Build history of the part. All positions in model axes, mm. Round coordinates to 2 decimals unless told otherwise and drop trailing zeros. Loops run counter-clockwise (first coordinate to the right, second up) from the corner with the lowest first, then second, coordinate; pieces in that order, holes last. Notation, with made-up numbers: (18, -37.75) -> (25, -37.75) arc R18 ccw to (25, -28.75) -> close; hole circle Ø9 at (36, 2.5). An arc over 180 degrees is marked (long way). Put each result on its own line as item: value. Start each with the question number.
```python
from build123d import *

# Parameters (mm, degrees)
SKETCH2_W           = 90
SKETCH2_H           = 94.61
SKETCH2_R           = 1.5
BOSS_EXTRUDE1_DEPTH = 3
SKETCH3_W           = 10.64
SKETCH3_H           = 65.81
CUT_EXTRUDE1_DEPTH  = 10
CHAMFER1_SIZE       = 2


with BuildPart() as part:
    # Sketch2 → Boss-Extrude1 (new body)
    with BuildSketch(Plane(origin=(0, 0, 0), x_dir=(1, 0, 0), z_dir=(0, 1, 0))):
        Rectangle(SKETCH2_W, SKETCH2_H)
        with Locations((40.082878696, -39.905)):
            Circle(SKETCH2_R, mode=Mode.SUBTRACT)
        with Locations((-40.357121304, -39.905)):
            Circle(SKETCH2_R, mode=Mode.SUBTRACT)
        with Locations((40.082878696, 40.095)):
            Circle(SKETCH2_R, mode=Mode.SUBTRACT)
        with Locations((-40.357121304, 40.095)):
            Circle(SKETCH2_R, mode=Mode.SUBTRACT)
    extrude(amount=BOSS_EXTRUDE1_DEPTH)

    # Sketch3 → Cut-Extrude1 (cut)
    with BuildSketch(Plane(origin=(0, 0, 0), x_dir=(-1, 0, 0), z_dir=(0, -1, 0))):
        with Locations((39.68, 0)):
            Rectangle(SKETCH3_W, SKETCH3_H)
        with Locations((-39.68, 0)):
            Rectangle(SKETCH3_W, SKETCH3_H)
    extrude(amount=-CUT_EXTRUDE1_DEPTH, mode=Mode.SUBTRACT)

    # Chamfer1
    chamfer1_edges = [part.edges().sort_by_distance(p)[0] for p in [
        (0, 0, -47.305),
    ]]
    chamfer(chamfer1_edges, length=CHAMFER1_SIZE)


solid = part.part
```
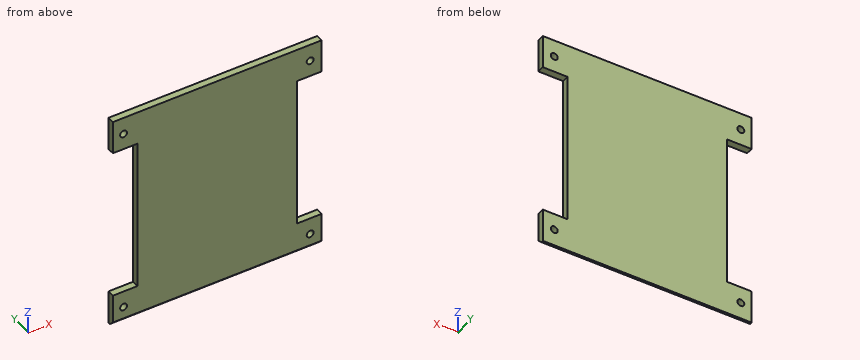
Item 1: Drop a flat-ended pin along its axis: pin 1 (1.5 mm diameter, centred on y = 2, z = 8, fed in from -X). Give the stop position or say it passes through.
Item 2: Cut at A-A on y = 0.9. Write the cut outline in (x, z) (3 decimals), then the cut area to 3 significant figures.
Item 3: Cut at B-B on z = -28.5. Write the cut outline in (x, y).
Item 4: Wall check: line 1 (Z direction, x = 35.5, y = 2.55) (3 decimals); line 2 (Z direction, x = 39, y = 1.15) (3 decimals); line 3 (X direction, y = 1.1, z = -41). Give the ranges that are in metal, low to high. Write a range as from..to.
Ans:
1. pin 1: stops at x = -34.36
2. outline: (-45, -46.205) -> (45, -46.205) -> (45, -32.905) -> (34.36, -32.905) -> (34.36, 32.905) -> (45, 32.905) -> (45, 47.305) -> (-45, 47.305) -> (-45, 32.905) -> (-34.36, 32.905) -> (-34.36, -32.905) -> (-45, -32.905) -> close; hole circle Ø3 at (-40.357, -40.095); hole circle Ø3 at (-40.357, 39.905); hole circle Ø3 at (40.083, -40.095); hole circle Ø3 at (40.083, 39.905)
2. area: 6,990 mm2
3. outline: (-34.36, 0) -> (34.36, 0) -> (34.36, 3) -> (-34.36, 3) -> close
4. line 1: z = -47.305..-32.905, 32.905..47.305
4. line 2: z = -46.455..-41.133, -39.057..-32.905, 32.905..38.867, 40.943..47.305
4. line 3: x = -45..-41.55, -39.16..38.89, 41.28..45
